from build123d import *

# Parameters (mm, degrees)
SKETCH1_R           = 1.75
SKETCH1_R_2         = 11
SKETCH1_R_3         = 1.5
BOSS_EXTRUDE1_DEPTH = 4


with BuildPart() as part:
    # Sketch1 → Boss-Extrude1 (new body)
    with BuildSketch(Plane.XY):
        with BuildLine():
            Line((-10, -12.489995997), (-10, -46.892440974))
            add(Edge.make_bspline(
                [(-10, -46.892440974), (-14.369218745, -46.490133027), (-28.167584564, -42.861139713), (-50.099896224, -30.060662438), (-86.961390459, -27.922716714), (-115.783330075, -30.807532602), (-114.008518426, 0)],
                knots=[0.072781672, 0.072781672, 0.072781672, 0.072781672, 0.171379313, 0.397323978, 0.628335943, 1, 1, 1, 1], degree=3))
            add(Edge.make_bspline(
                [(-10, 46.892440974), (-14.369218745, 46.490133027), (-28.167584564, 42.861139713), (-50.099896224, 30.060662438), (-86.961390459, 27.922716714), (-115.783330075, 30.807532602), (-114.008518426, 0)],
                knots=[0.072781672, 0.072781672, 0.072781672, 0.072781672, 0.171379313, 0.397323978, 0.628335943, 1, 1, 1, 1], degree=3))
            Line((-10, 46.892440974), (-10, 12.489995997))
            ThreePointArc((-10, 12.489995997), (-16, 0), (-10, -12.489995997))
        make_face()
        with Locations((-96.5, 15.5)):
            Circle(SKETCH1_R, mode=Mode.SUBTRACT)
        with Locations((-65.5, 15.5)):
            Circle(SKETCH1_R, mode=Mode.SUBTRACT)
        with Locations(Location((-65.5, -15.5, 0), (0, 0, 180))):
            Circle(SKETCH1_R, mode=Mode.SUBTRACT)
        with Locations(Location((-96.5, -15.5, 0), (0, 0, 180))):
            Circle(SKETCH1_R, mode=Mode.SUBTRACT)
        with Locations((-81, 0)):
            Circle(SKETCH1_R_2, mode=Mode.SUBTRACT)
        with Locations((-35.787805635, 0)):
            Circle(SKETCH1_R_3, mode=Mode.SUBTRACT)
        with Locations((-20, 20)):
            Circle(SKETCH1_R_3, mode=Mode.SUBTRACT)
        with Locations(Location((-20, -20, 0), (0, 0, 180))):
            Circle(SKETCH1_R_3, mode=Mode.SUBTRACT)
    extrude(amount=BOSS_EXTRUDE1_DEPTH)


solid = part.part
The model under review builds one solid part; all positions refer to its coordinate system, in mm. Round coordinates to 2 decimals unless told otherwise and drop trailing zeros. Use a Markdown table: item, result. Add a question column.
Q1. Insertion check: pin 1 (2 mm diameter, centred on y = -9, z = 0.5, fed in from -X); pin 2 (1.8 mm diameter, centred on x = -35.79, y = 0, fed in from -Z); pin 3 (1 mm diameter, centred on x = -78, z = 1, fed in from +Y); pin 4 (2 mm diameter, centred on y = -25.5, z = 2.5, fed in from -X). Each pin has a flat end and moves straight along its axis. Give the tip position at first contact, or say it passes through.
Q2. We need section A-A, the plane y = 15.5. Count the separate pieces of the cut face and the enclosed holes in it, plus the area to 3 significant figures.
Q3. To check wall thickness, follow line 1 (Y direction, x = -20, z = 3.1); line 2 (Y direction, x = -96.5, z = 2.1); line 3 (X direction, y = -15.5, z = 2.85). State the ranges of each line that lie inside material, in increasing order.
Q4. The part is to be moulded in two halves that separate along X. For faces 1 (the face through (-36.98, -0.91, 1.97)), 2 (the face through (-50, 1, 0)), 3 (the face through (-96.728, 17.235, 1.972)), 4 (the face through (-16, 0, 2)), say which applies: pulls with the +X half, pulls with the -X half, needs draft (parallel to the pull), parting line crosses it, or undercut.
Findings below:
| question | item | result |
|---|---|---|
| 1 | pin 1 | stops at x = -114 |
| 1 | pin 2 | passes through |
| 1 | pin 3 | stops at y = 28.95 |
| 1 | pin 4 | stops at x = -106.93 |
| 2 | separate pieces | 3 |
| 2 | enclosed holes | 0 |
| 2 | area | 383 mm² |
| 3 | line 1 | y = -44.82 to -21.5, -18.5 to 18.5, 21.5 to 44.82 |
| 3 | line 2 | y = -28.48 to -17.25, -13.75 to 13.75, 17.25 to 28.48 |
| 3 | line 3 | x = -112.7 to -98.25, -94.75 to -67.25, -63.75 to -10 |
| 4 | face 1 | undercut |
| 4 | face 2 | needs draft |
| 4 | face 3 | undercut |
| 4 | face 4 | pulls with the +X half |
